Answer from the drawing. Dimensions are ordinates in mm from the lowest x, y and z of the part. A direction names the side the tool comes from. Round coordinates to 2 decimals unless told otherwise and drop trailing zeros. Write each loop counter-clockwise with the first axis right and the second up, starting at its lowest first coordinate (ties: lowest second). Pieces come first, ordered by that corner, then holes. Notation, with made-up numbers: (-25, 7.5) - (16, 7.5) arc R38 cw to (16, 46.5) - close; hole circle Ø8 at (54, 19.25). An arc over 180 degrees is marked (long way). Return JSON: item names as keys, results as strings. Group by question number.
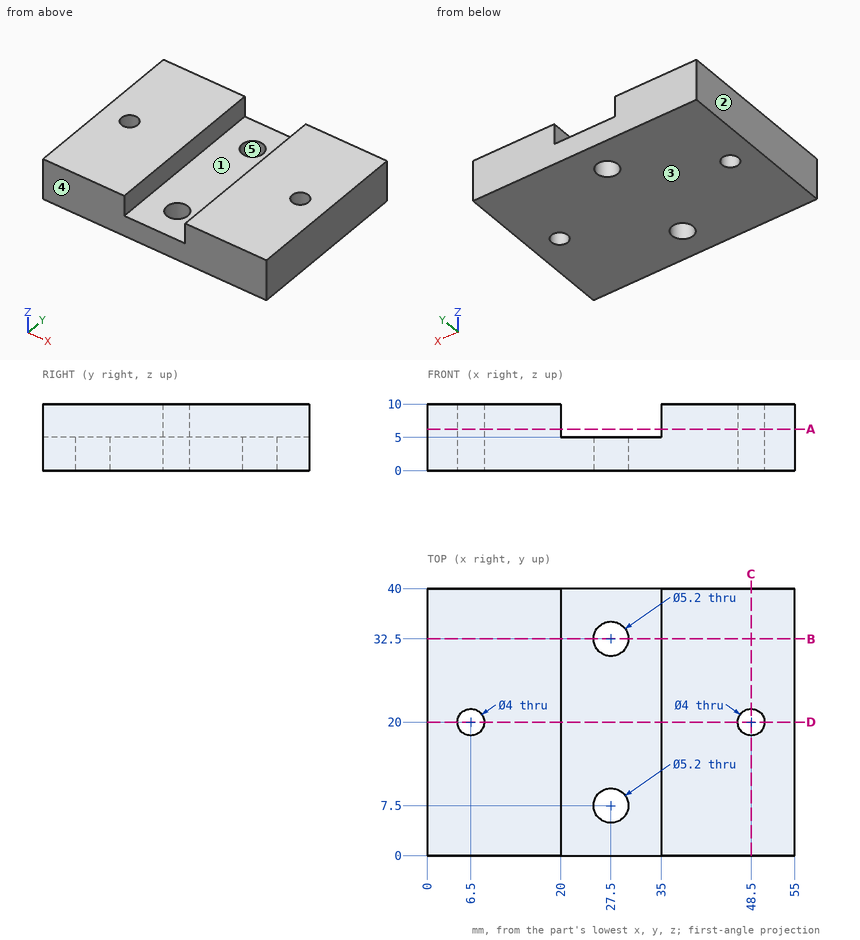
(1) Find section D-D (y = 20). Write down the section's boundary in (x, z).
(2) For the marked faces 1 and 2, determine the directions among +Z, -Z, +X, -X, +Y, -Y from which every point of the face is accessible in a straight line to the end or side of a thin tool.
(3) Find section A-A (z = 6.25). Write down the section's boundary in (x, y).
(4) Flat-ended cylindrical pins translate along their axes: pin 1 (7 mm diameter, centred on x = 27.5, y = 32.5, fed in from +Z); pin 2 (2.5 mm diameter, centred on x = 48.5, y = 20, fed in from -Z). Find the tip coordinate at first contact, or state that the pin passes through.
(5) Find section C-C (x = 48.5). Write down the section's boundary in (y, z).
(6) Consider line 1 (X direction, y = 20, z = 6); line 2 (X direction, y = 20, z = 4.25); line 3 (Y direction, x = 27.5, z = 3.6). Determine where each line is inside the solid, lowest interval first.
(7) Determine the mould class of the marked faces 3, 4 and 5 for opening direction Y: +Y half, -Y half, draft (parallel to the pull), parting line (faces both ways), or undercut.
(8) Find section B-B (y = 32.5). Write down the section's boundary in (x, z).
Check sheet entries:
{
 "1": {"outline": "(0, 0) - (4.5, 0) - (4.5, 10) - (0, 10) - close; (8.5, 0) - (46.5, 0) - (46.5, 10) - (35, 10) - (35, 5) - (20, 5) - (20, 10) - (8.5, 10) - close; (50.5, 0) - (55, 0) - (55, 10) - (50.5, 10) - close"},
 "2": {"face 1": "+Z, +Y, -Y", "face 2": "+Z, -Z, -X, +Y, -Y"},
 "3": {"outline": "(0, 0) - (20, 0) - (20, 40) - (0, 40) - close; (35, 0) - (55, 0) - (55, 40) - (35, 40) - close; hole circle Ø4 at (6.5, 20); hole circle Ø4 at (48.5, 20)"},
 "4": {"pin 1": "stops at z = 5", "pin 2": "passes through"},
 "5": {"outline": "(0, 0) - (18, 0) - (18, 10) - (0, 10) - close; (22, 0) - (40, 0) - (40, 10) - (22, 10) - close"},
 "6": {"line 1": "x = 0 to 4.5, 8.5 to 20, 35 to 46.5, 50.5 to 55", "line 2": "x = 0 to 4.5, 8.5 to 46.5, 50.5 to 55", "line 3": "y = 0 to 4.9, 10.1 to 29.9, 35.1 to 40"},
 "7": {"face 3": "draft", "face 4": "-Y half", "face 5": "undercut"},
 "8": {"outline": "(0, 0) - (24.9, 0) - (24.9, 5) - (20, 5) - (20, 10) - (0, 10) - close; (30.1, 0) - (55, 0) - (55, 10) - (35, 10) - (35, 5) - (30.1, 5) - close"}
}
